The listing builds one solid part. Answer for the finished solid, in the listing's coordinates (mm). Face numbers are marked on the shaded views. A direction names the side the tool comes from. Coordinates: 2 decimals unless noted, no trailing zeros. Order: outer loops, then holes, each group sorted by start corner. A loop starts at its lowest first (then second) coordinate and runs counter-clockwise, first axis right, second up. Notation, with made-up numbers: (-28, 85.25) - (31, 85.25) arc R16 cw to (31, 106.25) - close; hole circle Ø9 at (28.25, 53). An arc over 180 degrees is marked (long way). One line per item, written item: value. Start each with the question number.
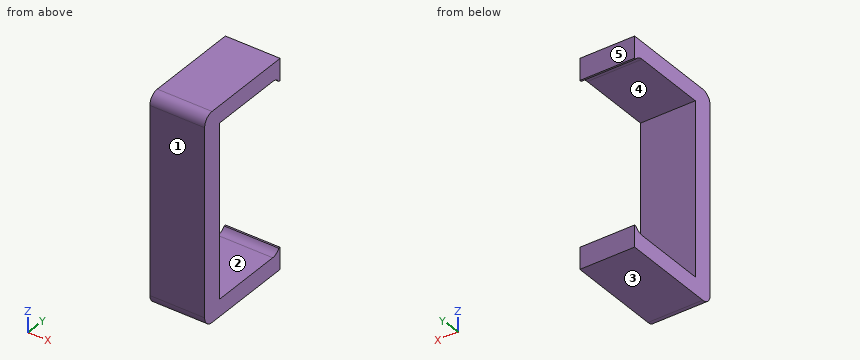
```python
from build123d import *

# Parameters (mm, degrees)
PROFILEBOSS_EXTRUDE1_DEPTH = 8


with BuildPart() as part:
    # Sketch2 → ProfileBoss-Extrude1 (new body)
    with BuildSketch(Plane(origin=(0, 0, 0), x_dir=(0, 0, -1), z_dir=(1, 0, 0))):
        with BuildLine():
            Line((1.5, 0), (28.75, 0))
            ThreePointArc((28.75, 0), (29.810660172, 0.439339828), (30.25, 1.5))
            Line((30.25, 1.5), (30.25, 15.25))
            Line((30.25, 15.25), (27.079156198, 15.25))
            Line((27.079156198, 15.25), (27.079156198, 15))
            ThreePointArc((27.079156198, 15), (27.571691018, 14.459318583), (27.75, 13.75))
            Line((27.75, 13.75), (27.75, 3))
            Line((27.75, 3), (2.5, 3))
            Line((2.5, 3), (2.5, 13.75))
            ThreePointArc((2.5, 13.75), (2.678308982, 14.459318583), (3.170843802, 15))
            Line((3.170843802, 15), (3.170843802, 15.25))
            Line((3.170843802, 15.25), (0, 15.25))
            Line((0, 15.25), (0, 1.5))
            ThreePointArc((0, 1.5), (0.439339828, 0.439339828), (1.5, 0))
        make_face()
    extrude(amount=PROFILEBOSS_EXTRUDE1_DEPTH)


solid = part.part
```
(1) The part is cut by section C-C on z = -15. Determine the outline of the cut face in (x, y).
(2) For the marked faces 4 and 5, determine the directions among +Z, -Z, +X, -X, +Y, -Y from which every point of the face is accessible in a straight line to the end or side of a thin tool.
(3) The part is cut by section B-B on x = 1.5. Determine the outline of the cut face in (y, z), plus the area to 3 significant figures.
(4) Consider probe 1 along Z at (x, y) = (0.75, 8.25); probe 2 along Y at (x, z) = (7, -12.5); probe 3 along Y at (x, z) = (5.25, -3). Determine where each line is inside the solid, lowest interval first.
(5) The part is cut by section A-A on y = 12.5. Determine the outline of the cut face in (x, z).
(6) For a pull along Y with two mould halves and no side action, classify the marked faces 1, 2 and 3 as pulls with the +Y half, pulls with the -Y half, needs draft (parallel to the pull), parting line crosses it, or undercut.
(7) A flat-ended cylindrical pin translates along its axis: pin 1 Ø2.5 at (x, z) = (5, -18.5) entering from +Y. Find the tip coordinate at first contact, or state that the pin passes through.
Completed:
1. outline: (0, 0) - (8, 0) - (8, 3) - (0, 3) - close
2. face 4: +X, -X
2. face 5: +Z, -Z, +X, -X, +Y
3. outline: (0, -28.75) arc R1.5 ccw to (1.5, -30.25) - (15.25, -30.25) - (15.25, -27.08) - (15, -27.08) arc R1.5 cw to (13.75, -27.75) - (3, -27.75) - (3, -2.5) - (13.75, -2.5) arc R1.5 cw to (15, -3.17) - (15.25, -3.17) - (15.25, 0) - (1.5, 0) arc R1.5 ccw to (0, -1.5) - close
3. area: 152 mm2
4. probe 1: z = -30.25 to -27.75, -2.5 to 0
4. probe 2: y = 0 to 3
4. probe 3: y = 0 to 3, 14.87 to 15.25
5. outline: (0, -30.25) - (8, -30.25) - (8, -27.75) - (0, -27.75) - close; (0, -2.5) - (8, -2.5) - (8, 0) - (0, 0) - close
6. face 1: pulls with the -Y half
6. face 2: undercut
6. face 3: needs draft
7. pin 1: stops at y = 3
